Source: CAD feature listing. Evaluate the final solid. Frame: model axes, mm. Face numbers are marked on the shaded views. Round coordinates to 2 decimals unless told otherwise and drop trailing zeros. Loops run counter-clockwise (first coordinate to the right, second up) from the corner with the lowest first, then second, coordinate; pieces in that order, holes last.
(1) Mould query, pull axis Z, two halves, no side actions, for the marked faces 1, 2 and 3. Classes: pulls with the +Z half, pulls with the -Z half, needs draft (parallel to the pull), parting line crosses it, or undercut.
(2) Section B-B, the plane z = -9. Return the cut outline in (x, y), plus the area to 3 significant figures.
(3) Material intervals for probe 1 along X at (y, z) = (2.45, 9.5); probe 2 along X at (y, z) = (1.2, -10); probe 3 along Z at (x, y) = (15.5, 0.45), sorted ascending.
(4) Section C-C, the plane y = 2.35. Return the cut outline in (x, z), plus the area to 3 significant figures.
(5) Section D-D, the plane z = 10. Return the cut outline in (x, y), plus the area to 3 significant figures.
(6) Section A-A, the plane x = 0. Return the cut outline in (y, z), plus the area to 3 significant figures.
(7) First-contact query: pin 1 Ø3 at (x, z) = (0, 10) entering from -Y; pin 2 Ø1.5 at (y, z) = (2, -10.5) entering from +X. Flat tips, straight axial feed; report the tip coordinate or a pass-through.
```python
from build123d import *

# Parameters (mm, degrees)
SKETCH1_W           = 50
SKETCH1_H           = 30
SKETCH1_R           = 1.75
SKETCH1_W_2         = 2.6
SKETCH1_H_2         = 8
BOSS_EXTRUDE2_DEPTH = 3
FILLET1_R           = 10


with BuildPart() as part:
    # Sketch1 → Boss-Extrude2 (new body)
    with BuildSketch(Plane(origin=(0, 0, 0), x_dir=(1, 0, 0), z_dir=(0, 1, 0))):
        Rectangle(SKETCH1_W, SKETCH1_H)
        with Locations(Location((-15, 10, 0), (0, 0, 270))):
            Circle(SKETCH1_R, mode=Mode.SUBTRACT)
        with Locations(Location((0, 10, 0), (0, 0, 270))):
            Circle(SKETCH1_R, mode=Mode.SUBTRACT)
        with Locations(Location((-15, -10, 0), (0, 0, 90))):
            Circle(SKETCH1_R, mode=Mode.SUBTRACT)
        with Locations(Location((0, -10, 0), (0, 0, 90))):
            Circle(SKETCH1_R, mode=Mode.SUBTRACT)
        with Locations((15, -9)):
            Rectangle(SKETCH1_W_2, SKETCH1_H_2, mode=Mode.SUBTRACT)
        with Locations((15, 9)):
            Rectangle(SKETCH1_W_2, SKETCH1_H_2, mode=Mode.SUBTRACT)
    extrude(amount=BOSS_EXTRUDE2_DEPTH)

    # Fillet1
    fillet1_edges = [part.edges().sort_by_distance(p)[0] for p in [
        (-25, 1.5, -15),
        (25, 1.5, -15),
        (25, 1.5, 15),
        (-25, 1.5, 15),
    ]]
    fillet(fillet1_edges, radius=FILLET1_R)


solid = part.part
```
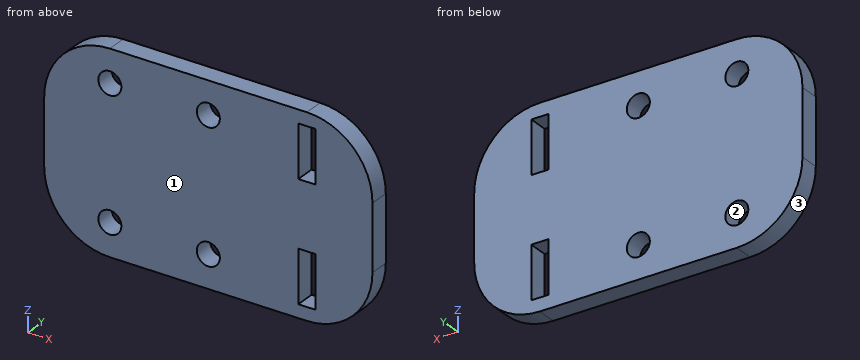
Output values:
1. face 1: needs draft
1. face 2: undercut
1. face 3: pulls with the -Z half
2. outline: (-24.17, 0) - (-16.44, 0) - (-16.44, 3) - (-24.17, 3) - close; (-13.56, 0) - (-1.44, 0) - (-1.44, 3) - (-13.56, 3) - close; (1.44, 0) - (13.7, 0) - (13.7, 3) - (1.44, 3) - close; (16.3, 0) - (24.17, 0) - (24.17, 3) - (16.3, 3) - close
2. area: 120 mm2
3. probe 1: x = -23.93 to -16.68, -13.32 to -1.68, 1.68 to 13.7, 16.3 to 23.93
3. probe 2: x = -23.66 to -16.75, -13.25 to -1.75, 1.75 to 13.7, 16.3 to 23.66
3. probe 3: z = -14.99 to -13, -5 to 5, 13 to 14.99
4. outline: (-25, -5) arc R10 ccw to (-15, -15) - (15, -15) arc R10 ccw to (25, -5) - (25, 5) arc R10 ccw to (15, 15) - (-15, 15) arc R10 ccw to (-25, 5) - close; hole circle Ø3.5 at (-15, -10); hole circle Ø3.5 at (-15, 10); hole circle Ø3.5 at (0, -10); hole circle Ø3.5 at (0, 10); hole (13.7, -13) - (16.3, -13) - (16.3, -5) - (13.7, -5) - close; hole (13.7, 5) - (16.3, 5) - (16.3, 13) - (13.7, 13) - close
4. area: 1,330 mm2
5. outline: (-23.66, 0) - (-16.75, 0) - (-16.75, 3) - (-23.66, 3) - close; (-13.25, 0) - (-1.75, 0) - (-1.75, 3) - (-13.25, 3) - close; (1.75, 0) - (13.7, 0) - (13.7, 3) - (1.75, 3) - close; (16.3, 0) - (23.66, 0) - (23.66, 3) - (16.3, 3) - close
5. area: 113 mm2
6. outline: (0, -15) - (3, -15) - (3, -11.75) - (0, -11.75) - close; (0, -8.25) - (3, -8.25) - (3, 8.25) - (0, 8.25) - close; (0, 11.75) - (3, 11.75) - (3, 15) - (0, 15) - close
6. area: 69.0 mm2
7. pin 1: passes through
7. pin 2: stops at x = 23.8
